Work out the finished part from the listing and answer in its coordinate system (mm). Coordinates: 2 decimals unless noted, no trailing zeros. Write each loop counter-clockwise with the first axis right and the second up, starting at its lowest first coordinate (ties: lowest second). Pieces come first, ordered by that corner, then holes. Notation, with made-up numbers: (68.5, -17.5) - (105.5, -17.5) arc R33 cw to (105.5, 14.5) - close; hole circle Ø8 at (9, -3). An arc over 180 degrees is marked (long way). Use one line per item in the form item = value. Start each with the question number.
Item 1: Consider probe 1 along Y at (x, z) = (-1395, 1.75); probe 2 along Y at (x, z) = (-1469, 1.4); probe 3 along Y at (x, z) = (-1424, 2.8). Determine where each line is inside the solid, lowest interval first.
Item 2: Given pin 1 (0.9 mm diameter, centred on x = -1425.5, z = 1, fed in from -Y), flat-ended and moving along its own axis, determine where the tip first touches the part or whether it passes through.
Item 3: A cutting plane is placed at B-B (x = -1418.5). Write down the section's boundary in (y, z), then the cut area to 3 significant figures.
Item 4: A cutting plane is placed at A-A (y = 288). Give the number of separate pieces and of enclosed holes in the cut face, then the cut area to 3 significant figures.
from build123d import *

# Parameters (mm, degrees)
MODEL_R                 = 1.5
SALIENTE_EXTRUIR1_DEPTH = 3


with BuildPart() as part:
    # Model → Saliente-Extruir1 (new body)
    with BuildSketch(Plane.XY):
        with BuildLine():
            Line((-1388.226934946, 304.407679238), (-1478.226934946, 304.407679238))
            ThreePointArc((-1478.226934946, 304.407679238), (-1481.408915461, 303.089659753), (-1482.726934946, 299.907679238))
            Line((-1482.726934946, 299.907679238), (-1482.726934946, 254.907679238))
            ThreePointArc((-1482.726934946, 254.907679238), (-1481.408915461, 251.725698722), (-1478.226934946, 250.407679238))
            Line((-1478.226934946, 250.407679238), (-1469.226934946, 250.407679238))
            ThreePointArc((-1469.226934946, 250.407679238), (-1466.04495443, 251.725698722), (-1464.726934946, 254.907679238))
            Line((-1464.726934946, 254.907679238), (-1464.726934946, 259.053577271))
            ThreePointArc((-1464.726934946, 259.053577271), (-1464.68680843, 259.398206652), (-1464.568575732, 259.724397665))
            Line((-1464.568575732, 259.724397665), (-1460.641524749, 267.578499631))
            ThreePointArc((-1460.641524749, 267.578499631), (-1460.088480631, 268.18365545), (-1459.299883963, 268.407679238))
            Line((-1459.299883963, 268.407679238), (-1407.153985929, 268.407679238))
            ThreePointArc((-1407.153985929, 268.407679238), (-1406.365389261, 268.18365545), (-1405.812345142, 267.578499631))
            Line((-1405.812345142, 267.578499631), (-1401.885294159, 259.724397665))
            ThreePointArc((-1401.885294159, 259.724397665), (-1401.767061462, 259.398206652), (-1401.726934946, 259.053577271))
            Line((-1401.726934946, 259.053577271), (-1401.726934946, 254.907679238))
            ThreePointArc((-1401.726934946, 254.907679238), (-1400.408915461, 251.725698722), (-1397.226934946, 250.407679238))
            Line((-1397.226934946, 250.407679238), (-1388.226934946, 250.407679238))
            ThreePointArc((-1388.226934946, 250.407679238), (-1385.04495443, 251.725698722), (-1383.726934946, 254.907679238))
            Line((-1383.726934946, 254.907679238), (-1383.726934946, 299.907679238))
            ThreePointArc((-1383.726934946, 299.907679238), (-1385.04495443, 303.089659753), (-1388.226934946, 304.407679238))
        make_face()
        with Locations((-1397.226934946, 254.907679238)):
            Circle(MODEL_R, mode=Mode.SUBTRACT)
        with Locations((-1397.226934946, 299.907679238)):
            Circle(MODEL_R, mode=Mode.SUBTRACT)
        with Locations((-1469.226934946, 254.907679238)):
            Circle(MODEL_R, mode=Mode.SUBTRACT)
        with Locations((-1424.226934946, 299.907679238)):
            Circle(MODEL_R, mode=Mode.SUBTRACT)
        with Locations((-1433.226934946, 299.907679238)):
            Circle(MODEL_R, mode=Mode.SUBTRACT)
        with Locations((-1442.226934946, 299.907679238)):
            Circle(MODEL_R, mode=Mode.SUBTRACT)
        with Locations((-1469.226934946, 299.907679238)):
            Circle(MODEL_R, mode=Mode.SUBTRACT)
        with Locations((-1478.226934946, 254.907679238)):
            Circle(MODEL_R, mode=Mode.SUBTRACT)
        with Locations((-1478.226934946, 299.907679238)):
            Circle(MODEL_R, mode=Mode.SUBTRACT)
        with Locations((-1388.226934946, 254.907679238)):
            Circle(MODEL_R, mode=Mode.SUBTRACT)
        with Locations((-1388.226934946, 299.907679238)):
            Circle(MODEL_R, mode=Mode.SUBTRACT)
        with Locations((-1406.226934946, 272.907679238)):
            Circle(MODEL_R, mode=Mode.SUBTRACT)
        with Locations((-1415.226934946, 272.907679238)):
            Circle(MODEL_R, mode=Mode.SUBTRACT)
        with Locations((-1424.226934946, 272.907679238)):
            Circle(MODEL_R, mode=Mode.SUBTRACT)
        with Locations((-1433.226934946, 272.907679238)):
            Circle(MODEL_R, mode=Mode.SUBTRACT)
        with Locations((-1442.226934946, 272.907679238)):
            Circle(MODEL_R, mode=Mode.SUBTRACT)
        with Locations((-1451.226934946, 272.907679238)):
            Circle(MODEL_R, mode=Mode.SUBTRACT)
        with Locations((-1460.226934946, 272.907679238)):
            Circle(MODEL_R, mode=Mode.SUBTRACT)
        with BuildLine():
            Line((-1458.726934946, 281.907679238), (-1458.726934946, 290.907679238))
            ThreePointArc((-1458.726934946, 290.907679238), (-1460.226934946, 292.407679238), (-1461.726934946, 290.907679238))
            Line((-1461.726934946, 290.907679238), (-1461.726934946, 281.907679238))
            ThreePointArc((-1461.726934946, 281.907679238), (-1460.226934946, 280.407679238), (-1458.726934946, 281.907679238))
        make_face(mode=Mode.SUBTRACT)
        with BuildLine():
            Line((-1449.726934946, 281.907679238), (-1449.726934946, 290.907679238))
            ThreePointArc((-1449.726934946, 290.907679238), (-1451.226934946, 292.407679238), (-1452.726934946, 290.907679238))
            Line((-1452.726934946, 290.907679238), (-1452.726934946, 281.907679238))
            ThreePointArc((-1452.726934946, 281.907679238), (-1451.226934946, 280.407679238), (-1449.726934946, 281.907679238))
        make_face(mode=Mode.SUBTRACT)
        with BuildLine():
            Line((-1440.726934946, 281.907679238), (-1440.726934946, 290.907679238))
            ThreePointArc((-1440.726934946, 290.907679238), (-1442.226934946, 292.407679238), (-1443.726934946, 290.907679238))
            Line((-1443.726934946, 290.907679238), (-1443.726934946, 281.907679238))
            ThreePointArc((-1443.726934946, 281.907679238), (-1442.226934946, 280.407679238), (-1440.726934946, 281.907679238))
        make_face(mode=Mode.SUBTRACT)
        with BuildLine():
            Line((-1431.726934946, 281.907679238), (-1431.726934946, 290.907679238))
            ThreePointArc((-1431.726934946, 290.907679238), (-1433.226934946, 292.407679238), (-1434.726934946, 290.907679238))
            Line((-1434.726934946, 290.907679238), (-1434.726934946, 281.907679238))
            ThreePointArc((-1434.726934946, 281.907679238), (-1433.226934946, 280.407679238), (-1431.726934946, 281.907679238))
        make_face(mode=Mode.SUBTRACT)
        with BuildLine():
            Line((-1422.726934946, 281.907679238), (-1422.726934946, 290.907679238))
            ThreePointArc((-1422.726934946, 290.907679238), (-1424.226934946, 292.407679238), (-1425.726934946, 290.907679238))
            Line((-1425.726934946, 290.907679238), (-1425.726934946, 281.907679238))
            ThreePointArc((-1425.726934946, 281.907679238), (-1424.226934946, 280.407679238), (-1422.726934946, 281.907679238))
        make_face(mode=Mode.SUBTRACT)
        with BuildLine():
            Line((-1413.726934946, 281.907679238), (-1413.726934946, 290.907679238))
            ThreePointArc((-1413.726934946, 290.907679238), (-1415.226934946, 292.407679238), (-1416.726934946, 290.907679238))
            Line((-1416.726934946, 290.907679238), (-1416.726934946, 281.907679238))
            ThreePointArc((-1416.726934946, 281.907679238), (-1415.226934946, 280.407679238), (-1413.726934946, 281.907679238))
        make_face(mode=Mode.SUBTRACT)
        with BuildLine():
            Line((-1404.726934946, 281.907679238), (-1404.726934946, 290.907679238))
            ThreePointArc((-1404.726934946, 290.907679238), (-1406.226934946, 292.407679238), (-1407.726934946, 290.907679238))
            Line((-1407.726934946, 290.907679238), (-1407.726934946, 281.907679238))
            ThreePointArc((-1407.726934946, 281.907679238), (-1406.226934946, 280.407679238), (-1404.726934946, 281.907679238))
        make_face(mode=Mode.SUBTRACT)
        with BuildLine():
            Line((-1478.226934946, 292.407679238), (-1469.226934946, 292.407679238))
            ThreePointArc((-1469.226934946, 292.407679238), (-1467.726934946, 290.907679238), (-1469.226934946, 289.407679238))
            Line((-1469.226934946, 289.407679238), (-1478.226934946, 289.407679238))
            ThreePointArc((-1478.226934946, 289.407679238), (-1479.726934946, 290.907679238), (-1478.226934946, 292.407679238))
        make_face(mode=Mode.SUBTRACT)
        with BuildLine():
            Line((-1397.226934946, 292.407679238), (-1388.226934946, 292.407679238))
            ThreePointArc((-1388.226934946, 292.407679238), (-1386.726934946, 290.907679238), (-1388.226934946, 289.407679238))
            Line((-1388.226934946, 289.407679238), (-1397.226934946, 289.407679238))
            ThreePointArc((-1397.226934946, 289.407679238), (-1398.726934946, 290.907679238), (-1397.226934946, 292.407679238))
        make_face(mode=Mode.SUBTRACT)
        with BuildLine():
            Line((-1397.226934946, 280.407679238), (-1388.226934946, 280.407679238))
            ThreePointArc((-1388.226934946, 280.407679238), (-1386.726934946, 281.907679238), (-1388.226934946, 283.407679238))
            Line((-1388.226934946, 283.407679238), (-1397.226934946, 283.407679238))
            ThreePointArc((-1397.226934946, 283.407679238), (-1398.726934946, 281.907679238), (-1397.226934946, 280.407679238))
        make_face(mode=Mode.SUBTRACT)
        with BuildLine():
            Line((-1460.226934946, 298.407679238), (-1451.226934946, 298.407679238))
            ThreePointArc((-1451.226934946, 298.407679238), (-1449.726934946, 299.907679238), (-1451.226934946, 301.407679238))
            Line((-1451.226934946, 301.407679238), (-1460.226934946, 301.407679238))
            ThreePointArc((-1460.226934946, 301.407679238), (-1461.726934946, 299.907679238), (-1460.226934946, 298.407679238))
        make_face(mode=Mode.SUBTRACT)
        with BuildLine():
            Line((-1415.226934946, 301.407679238), (-1406.226934946, 301.407679238))
            ThreePointArc((-1406.226934946, 301.407679238), (-1404.726934946, 299.907679238), (-1406.226934946, 298.407679238))
            Line((-1406.226934946, 298.407679238), (-1415.226934946, 298.407679238))
            ThreePointArc((-1415.226934946, 298.407679238), (-1416.726934946, 299.907679238), (-1415.226934946, 301.407679238))
        make_face(mode=Mode.SUBTRACT)
        with BuildLine():
            Line((-1478.226934946, 280.407679238), (-1469.226934946, 280.407679238))
            ThreePointArc((-1469.226934946, 280.407679238), (-1467.726934946, 281.907679238), (-1469.226934946, 283.407679238))
            Line((-1469.226934946, 283.407679238), (-1478.226934946, 283.407679238))
            ThreePointArc((-1478.226934946, 283.407679238), (-1479.726934946, 281.907679238), (-1478.226934946, 280.407679238))
        make_face(mode=Mode.SUBTRACT)
    extrude(amount=SALIENTE_EXTRUIR1_DEPTH)


solid = part.part
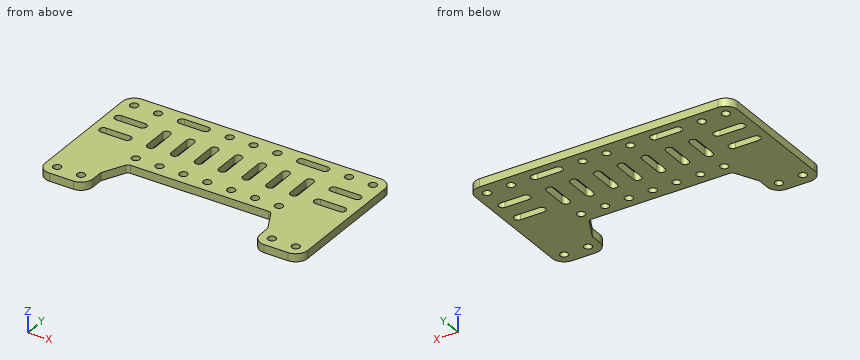
Answer:
q1.probe_1 = 250.41 to 280.41, 283.41 to 289.41, 292.41 to 304.41
q1.probe_2 = 250.41 to 253.42, 256.39 to 280.42, 283.39 to 289.42, 292.39 to 298.42, 301.39 to 304.41
q1.probe_3 = 268.41 to 271.42, 274.39 to 280.42, 292.39 to 298.42, 301.39 to 304.41
q2.pin_1 = 268.41
q3.outline = (268.41, 0) - (304.41, 0) - (304.41, 3) - (268.41, 3) - close
q3.area = 108 mm²
q4.separate_pieces = 8
q4.enclosed_holes = 0
q4.area = 234 mm²
